Design review of the part built by this model. Coordinates are the model's own, in mm. A direction names the side the tool comes from. Give positions to 0.01 mm unless a question says otherwise; leave off trailing zeros. Order: outer loops, then holes, each group sorted by start corner. A loop starts at its lowest first (then second) coordinate and runs counter-clockwise, first axis right, second up.
```python
from build123d import *

# Parameters (mm, degrees)
CYLINDER235_R          = 4.2
CYLINDER235_DEPTH      = 18
CYLINDER235_ROLL_ANGLE = 90
CYLINDER237_R          = 1.7
CYLINDER237_DEPTH      = 20
CYLINDER237_ROLL_ANGLE = 90
CYLINDER236_R          = 1.7
CYLINDER236_DEPTH      = 20
CYLINDER236_ROLL_ANGLE = 90
BOX001027045178_W      = 10
BOX001027045178_H      = 4
BOX001027045178_DEPTH  = 60
CYLINDER234_R          = 2
CYLINDER234_DEPTH      = 74
BOX001027045177_W      = 16
BOX001027045177_H      = 4.5
BOX001027045177_DEPTH  = 20


with BuildPart() as rocker_cut004:
    # Cylinder235 → Cylinder235 (new body)
    with BuildSketch(Plane.XY):
        Circle(CYLINDER235_R)
    extrude(amount=CYLINDER235_DEPTH)


with BuildPart() as rocker_cut004_1:
    # Cylinder235 roll: moved
    add(rocker_cut004.part.rotate(Axis((0, 0, 0), (1, 0, 0)), CYLINDER235_ROLL_ANGLE))


with BuildPart() as rocker_cut004_2:
    # Cylinder235 placement: moved
    add(rocker_cut004_1.part.moved(Location((0, 9, -8))))


with BuildPart() as cylinder264:
    # Cylinder237 → Cylinder237 (new body)
    with BuildSketch(Plane.XY):
        Circle(CYLINDER237_R)
    extrude(amount=CYLINDER237_DEPTH)


with BuildPart() as cylinder264_1:
    # Cylinder237 roll: moved
    add(cylinder264.part.rotate(Axis((0, 0, 0), (1, 0, 0)), CYLINDER237_ROLL_ANGLE))


with BuildPart() as cylinder264_2:
    # Cylinder237 placement: moved
    add(cylinder264_1.part.moved(Location((7, 11, -13))))


with BuildPart() as top_slot_m3_clearance001:
    # Cylinder236 → Cylinder236 (new body)
    with BuildSketch(Plane.XY):
        Circle(CYLINDER236_R)
    extrude(amount=CYLINDER236_DEPTH)


with BuildPart() as top_slot_m3_clearance001_1:
    # Cylinder236 roll: moved
    add(top_slot_m3_clearance001.part.rotate(Axis((0, 0, 0), (1, 0, 0)), CYLINDER236_ROLL_ANGLE))


with BuildPart() as top_slot_m3_clearance001_2:
    # Cylinder236 placement: moved
    add(top_slot_m3_clearance001_1.part.moved(Location((7, 11, -26))))

    # Fusion112126: union Cylinder264
    add(cylinder264_2.part)


with BuildPart() as cube226:
    # Box001027045178 → Box001027045178 (new body)
    with BuildSketch(Plane(origin=(-10, -2, -57), x_dir=(1, 0, 0), z_dir=(0, 0, 1))):
        with Locations((5, 2)):
            Rectangle(BOX001027045178_W, BOX001027045178_H)
    extrude(amount=BOX001027045178_DEPTH)


with BuildPart() as plate_cuts:
    # Cylinder234 → Cylinder234 (new body)
    with BuildSketch(Plane.XY.offset(-62)):
        Circle(CYLINDER234_R)
    extrude(amount=CYLINDER234_DEPTH)

    # Fusion112125: union Cube226
    add(cube226.part)


with BuildPart() as plate_cuts_1:
    # Fusion112125 placement: moved
    add(plate_cuts.part.moved(Location((2.5, 0, 0))))

    # Fusion112127: union rocker-cut004, top-slot-m3-clearance001
    add(rocker_cut004_2.part)
    add(top_slot_m3_clearance001_2.part)


with BuildPart() as top_slot_plate:
    # Box001027045177 → Box001027045177 (new body)
    with BuildSketch(Plane(origin=(-5, 0, -30), x_dir=(1, 0, 0), z_dir=(0, 0, 1))):
        with Locations((8, 2.25)):
            Rectangle(BOX001027045177_W, BOX001027045177_H)
    extrude(amount=BOX001027045177_DEPTH)

    # Cut217: cut plate-cuts
    add(plate_cuts_1.part, mode=Mode.SUBTRACT)


solid = top_slot_plate.part
```
1. Take a section at B-B (y = 4.2). State the section outline as (x, z) points, then the cut area to 3 significant figures.
Recorded:
outline: (-5, -30) - (11, -30) - (11, -10) - (3.69, -10) arc R4.2 cw to (-3.69, -10) - (-5, -10) - close; hole circle Ø3.4 at (7, -26); hole circle Ø3.4 at (7, -13)
area: 290 mm2
2. Take a section at C-C (z = -26). State the section outline as (x, y) points.
Recorded:
outline: (-5, 2) - (2.5, 2) arc R2 cw to (4.5, 0) - (5.3, 0) - (5.3, 4.5) - (-5, 4.5) - close; (8.7, 0) - (11, 0) - (11, 4.5) - (8.7, 4.5) - close
3. Draft analysis for pull direction Z (two halves, no side actions). For faces 3 (the face through (5, 3, -30)), 4 (the face through (3, 4.5, -20)), 5 (the face through (-4, 3, -10)), 6 (the face through (5.75, 2.28, -11.85)), state which applies: pulls with the +Z half, pulls with the -Z half, needs draft (parallel to the pull), parting line crosses it, or undercut.
Recorded:
face 3: pulls with the -Z half
face 4: needs draft
face 5: pulls with the +Z half
face 6: undercut
4. Machinability: for faces 1 (the face through (7, 2, -10)), 2 (the face through (-1, 2, -20)), which of the approach directions +Z, -Z, +X, -X, +Y, -Y give a long, thin tool a straight path to every point of the face, cutting with its end or side? Answer none if there is none.
Recorded:
face 1: +Z, +X, -X, +Y, -Y
face 2: +Z, -Z, -X, -Y
5. Take a section at A-A (x = 7). State the section outline as (y, z) points, then the cut area to 3 significant figures.
Recorded:
outline: (0, -30) - (4.5, -30) - (4.5, -27.7) - (0, -27.7) - close; (0, -24.3) - (4.5, -24.3) - (4.5, -14.7) - (0, -14.7) - close; (0, -11.3) - (4.5, -11.3) - (4.5, -10) - (0, -10) - close
area: 59.4 mm2
6. For pin 1 (4 mm diameter, centred on x = 0, z = -20.5, fed in from -Y), flat-tipped, find the tip position at first contact; note if it passes through.
Recorded:
pin 1: stops at y = 2
7. Take a section at D-D (z = -21.5). State the section outline as (x, y) points.
Recorded:
outline: (-5, 2) - (2.5, 2) arc R2 cw to (4.5, 0) - (11, 0) - (11, 4.5) - (-5, 4.5) - close
8. For line 1 along Z through (x, y) = (7, 3.5); line 2 along Z through (x, y) = (5.5, 4.05); line 3 along X through (y, z) = (1.65, -13), list the stretches that pass through material, from the lowest coordinate up.
Recorded:
line 1: z = -30 to -27.7, -24.3 to -14.7, -11.3 to -10
line 2: z = -30 to -26.8, -25.2 to -13.8, -12.2 to -10
line 3: x = 3.63 to 5.3, 8.7 to 11
